from build123d import *

# Parameters (mm, degrees)
BOSS_EXTRUDE1_DEPTH     = 20.2
BOSS_EXTRUDE3_DEPTH     = 130
SKETCH7_R               = 4.5
CUT_EXTRUDE1_DEPTH      = 10
CUT_EXTRUDE2_DEPTH      = 119.099419302
CUT_EXTRUDE2_DEPTH_BACK = 119.099419302
SKETCH8_W               = 3
SKETCH8_H               = 58.2


with BuildPart() as part:
    # Sketch1 → Boss-Extrude1 (new body)
    with BuildSketch(Plane.XY):
        Polygon((-76.580441788, 84.160209426), (-76.580441788, 48.260209426), (-73.580441788, 48.260209426), (-73.580441788, -9.939790574), (-76.580441788, -9.939790574), (-76.580441788, -45.839790574), (-72.580441788, -45.839790574), (-72.580441788, 84.160209426), align=None)
    extrude(amount=BOSS_EXTRUDE1_DEPTH)

    # Sketch2 → Boss-Extrude3 (add)
    with BuildSketch(Plane(origin=(0, 84.160209426, 0), x_dir=(1, 0, 0), z_dir=(0, 1, 0))):
        with BuildLine():
            Line((-72.580441788, -20.2), (-76.580441788, -20.2))
            ThreePointArc((-76.580441788, -20.2), (-67.602885827, -29.171952003), (-55.120441788, -31.47))
            Line((-55.120441788, -31.47), (-55.120441788, -27.56))
            ThreePointArc((-55.120441788, -27.56), (-63.136226216, -25.611247532), (-69.362688802, -20.2))
            Line((-69.362688802, -20.2), (-72.580441788, -20.2))
        make_face()
        with BuildLine():
            Line((-76.580441788, 0), (-72.580441788, 0))
            Line((-72.580441788, 0), (-69.362688802, 0))
            ThreePointArc((-69.362688802, 0), (-63.136226216, 5.411247532), (-55.120441788, 7.36))
            Line((-55.120441788, 7.36), (-55.120441788, 11.27))
            ThreePointArc((-55.120441788, 11.27), (-67.602885827, 8.971952003), (-76.580441788, 0))
        make_face()
        with BuildLine():
            Line((-69.362688802, 0), (-72.580441788, 0))
            Line((-72.580441788, 0), (-72.580441788, -10.1))
            ThreePointArc((-72.580441788, -10.1), (-71.756565628, -4.799907211), (-69.362688802, 0))
        make_face()
        with BuildLine():
            ThreePointArc((-69.362688802, -20.2), (-71.756565628, -15.400092789), (-72.580441788, -10.1))
            Line((-72.580441788, -10.1), (-72.580441788, -20.2))
            Line((-72.580441788, -20.2), (-69.362688802, -20.2))
        make_face()
    extrude(amount=-BOSS_EXTRUDE3_DEPTH)

    # Sketch7 → Cut-Extrude1 (cut)
    with BuildSketch(Plane.ZY.offset(76.580441788)):
        with Locations(Location((10.1, 69.160209426, 0), (0, 0, 270))):
            Circle(SKETCH7_R)
        with Locations(Location((10.1, 34.160209426, 0), (0, 0, 270))):
            Circle(SKETCH7_R)
        with Locations(Location((10.1, -0.839790574, 0), (0, 0, 270))):
            Circle(SKETCH7_R)
        with Locations(Location((10.1, -35.839790574, 0), (0, 0, 270))):
            Circle(SKETCH7_R)
    extrude(amount=-CUT_EXTRUDE1_DEPTH, mode=Mode.SUBTRACT)

    # Sketch8 → Cut-Extrude2 (cut, two sides: drawn at the far end of the back side and taken through both)
    with BuildSketch(Plane.XY.offset(-CUT_EXTRUDE2_DEPTH_BACK)):
        with Locations((-75.080441788, 19.160209426)):
            Rectangle(SKETCH8_W, SKETCH8_H)
    extrude(amount=CUT_EXTRUDE2_DEPTH + CUT_EXTRUDE2_DEPTH_BACK, mode=Mode.SUBTRACT)


solid = part.part
The model under review builds one solid part; all positions refer to its coordinate system, in mm. A direction names the side the tool comes from. Round coordinates to 2 decimals unless told otherwise and drop trailing zeros. Write each loop counter-clockwise with the first axis right and the second up, starting at its lowest first coordinate (ties: lowest second). Pieces come first, ordered by that corner, then holes. Notation, with made-up numbers: (53.5, 22) -> (100.5, 22) arc R19 cw to (100.5, 52) -> close; hole circle Ø11 at (-13.5, 65). An arc over 180 degrees is marked (long way). Answer as a JSON object with one key per item and string values.
1. We need section D-D on z = 23. State the section outline as (x, y) points.
Results found:
{"outline": "(-74.82, -45.84) -> (-66.89, -45.84) -> (-66.89, 84.16) -> (-74.82, 84.16) -> (-74.82, 48.26) -> (-73.58, 48.26) -> (-73.58, -9.94) -> (-74.82, -9.94) -> close"}
2. We need section A-A on y = 66.5. State the section outline as (x, z) points, and give its area (3 significant figures).
Results found:
{"outline": "(-76.58, 0) arc R21.37 ccw to (-55.12, -11.27) -> (-55.12, -7.36) arc R17.46 cw to (-72.2, 6.47) -> (-76.58, 6.47) -> close; (-76.58, 13.73) -> (-72.2, 13.73) arc R17.46 cw to (-55.12, 27.56) -> (-55.12, 31.47) arc R21.37 ccw to (-76.58, 20.2) -> close", "area": "291 mm^2"}
3. To check wall thickness, follow line 1 along Y through (x, z) = (-75.3, 10.1); line 2 along Y through (x, z) = (-72.8, 10.1); line 3 along Y through (x, z) = (-74.5, 12). State the ranges of each line that lie inside material, in increasing order.
Results found:
{"line 1": "y = -45.84 to -40.34, -31.34 to -9.94, 48.26 to 64.66, 73.66 to 84.16", "line 2": "y = -45.84 to -40.34, -31.34 to -5.34, 3.66 to 29.66, 38.66 to 64.66, 73.66 to 84.16", "line 3": "y = -45.84 to -39.92, -31.76 to -9.94, 48.26 to 65.08, 73.24 to 84.16"}
4. We need section C-C on z = 12. State the section outline as (x, y) points, and give its area (3 significant figures).
Results found:
{"outline": "(-76.58, -45.84) -> (-72.48, -45.84) -> (-72.48, -39.92) -> (-76.58, -39.92) -> close; (-76.58, -31.76) -> (-72.48, -31.76) -> (-72.48, -4.92) -> (-73.58, -4.92) -> (-73.58, -9.94) -> (-76.58, -9.94) -> close; (-76.58, 48.26) -> (-73.58, 48.26) -> (-73.58, 38.24) -> (-72.48, 38.24) -> (-72.48, 65.08) -> (-76.58, 65.08) -> close; (-76.58, 73.24) -> (-72.48, 73.24) -> (-72.48, 84.16) -> (-76.58, 84.16) -> close; (-73.58, 3.24) -> (-72.48, 3.24) -> (-72.48, 30.08) -> (-73.58, 30.08) -> close", "area": "274 mm^2"}
5. The part is to be moulded in two halves that separate along Z. For faces 1 (the face through (-55.12, 20, -9)), 2 (the face through (-67.443, 20.07, -9.055)), 3 (the face through (-72.973, 38.656, 10.298)), say which applies: pulls with the +Z half, pulls with the -Z half, needs draft (parallel to the pull), parting line crosses it, or undercut.
Results found:
{"face 1": "needs draft", "face 2": "pulls with the -Z half", "face 3": "undercut"}
6. We need section B-B on x = -68. State the section outline as (y, z) points.
Results found:
{"outline": "(-45.84, -8.76) -> (84.16, -8.76) -> (84.16, -1.69) -> (-45.84, -1.69) -> close; (-45.84, 21.89) -> (84.16, 21.89) -> (84.16, 28.96) -> (-45.84, 28.96) -> close"}
7. Machinability: for faces 4 (the face through (-74.318, -40.132, 11.452)), 5 (the face through (-73.58, 19, 10)), which of the approach directions +Z, -Z, +X, -X, +Y, -Y give a long, thin tool a straight path to every point of the face, cutting with its end or side? Answer none if there is none.
Results found:
{"face 4": "+X, -X", "face 5": "+Z, -Z, -X"}
8. Clearance check with flat-ended pins moving along their axes: pin 1 (11.5 mm diameter, centred on y = 69.16, z = 10.1, fed in from +X); pin 2 (1 mm diameter, centred on y = 37.5, z = 15, fed in from -X); pin 3 (5.5 mm diameter, centred on y = -35.84, z = 10.1, fed in from -X); pin 4 (1 mm diameter, centred on x = -74, y = 13.5, fed in from +Z). State where each tip first meets the part, or that it passes through.
Results found:
{"pin 1": "stops at x = -71.61", "pin 2": "stops at x = -73.58", "pin 3": "passes through", "pin 4": "stops at z = 24.6"}
